from build123d import *

# Parameters (mm, degrees)
ESBO_O1_W                = 231.5
ESBO_O1_H                = 170
RESSALTO_EXTRUS_O1_DEPTH = 3
CORTE_EXTRUS_O1_REACH    = 145.639
ESBO_O2_W                = 17.807692308
ESBO_O2_H                = 6
CORTE_EXTRUS_O2_REACH    = 145.639
ESBO_O3_W                = 6
ESBO_O3_H                = 15.454545455


with BuildPart() as part:
    # Esboço1 → Ressalto-extrusão1 (new body)
    with BuildSketch(Plane(origin=(0, 0, 0), x_dir=(1, 0, 0), z_dir=(0, 1, 0))):
        Rectangle(ESBO_O1_W, ESBO_O1_H)
    extrude(amount=RESSALTO_EXTRUS_O1_DEPTH)

    # Esboço2 → Corte-extrusão1 (cut, up to next)
    with BuildSketch(Plane.XZ, mode=Mode.PRIVATE) as corte_extrus_o1_sk1:
        with Locations((-71.226153846, 82)):
            Rectangle(ESBO_O2_W, ESBO_O2_H)
    corte_extrus_o1_tool1 = extrude(corte_extrus_o1_sk1.sketch, amount=-CORTE_EXTRUS_O1_REACH, mode=Mode.PRIVATE) & part.part
    # Esboço2 → Corte-extrusão1 (cut, up to next)
    with BuildSketch(Plane.XZ, mode=Mode.PRIVATE) as corte_extrus_o1_sk2:
        with Locations((-106.846153846, 82)):
            Rectangle(ESBO_O2_W, ESBO_O2_H)
    corte_extrus_o1_tool2 = extrude(corte_extrus_o1_sk2.sketch, amount=-CORTE_EXTRUS_O1_REACH, mode=Mode.PRIVATE) & part.part
    # Esboço2 → Corte-extrusão1 (cut, up to next)
    with BuildSketch(Plane.XZ, mode=Mode.PRIVATE) as corte_extrus_o1_sk3:
        with Locations((-35.606153846, 82)):
            Rectangle(ESBO_O2_W, ESBO_O2_H)
    corte_extrus_o1_tool3 = extrude(corte_extrus_o1_sk3.sketch, amount=-CORTE_EXTRUS_O1_REACH, mode=Mode.PRIVATE) & part.part
    # Esboço2 → Corte-extrusão1 (cut, up to next)
    with BuildSketch(Plane.XZ, mode=Mode.PRIVATE) as corte_extrus_o1_sk4:
        with Locations((0.013846154, 82)):
            Rectangle(ESBO_O2_W, ESBO_O2_H)
    corte_extrus_o1_tool4 = extrude(corte_extrus_o1_sk4.sketch, amount=-CORTE_EXTRUS_O1_REACH, mode=Mode.PRIVATE) & part.part
    # Esboço2 → Corte-extrusão1 (cut, up to next)
    with BuildSketch(Plane.XZ, mode=Mode.PRIVATE) as corte_extrus_o1_sk5:
        with Locations((35.633846154, 82)):
            Rectangle(ESBO_O2_W, ESBO_O2_H)
    corte_extrus_o1_tool5 = extrude(corte_extrus_o1_sk5.sketch, amount=-CORTE_EXTRUS_O1_REACH, mode=Mode.PRIVATE) & part.part
    # Esboço2 → Corte-extrusão1 (cut, up to next)
    with BuildSketch(Plane.XZ, mode=Mode.PRIVATE) as corte_extrus_o1_sk6:
        with Locations((71.253846154, 82)):
            Rectangle(ESBO_O2_W, ESBO_O2_H)
    corte_extrus_o1_tool6 = extrude(corte_extrus_o1_sk6.sketch, amount=-CORTE_EXTRUS_O1_REACH, mode=Mode.PRIVATE) & part.part
    # Esboço2 → Corte-extrusão1 (cut, up to next)
    with BuildSketch(Plane.XZ, mode=Mode.PRIVATE) as corte_extrus_o1_sk7:
        with Locations((106.873846154, 82)):
            Rectangle(ESBO_O2_W, ESBO_O2_H)
    corte_extrus_o1_tool7 = extrude(corte_extrus_o1_sk7.sketch, amount=-CORTE_EXTRUS_O1_REACH, mode=Mode.PRIVATE) & part.part
    # Esboço2 → Corte-extrusão1 (cut, up to next)
    with BuildSketch(Plane.XZ, mode=Mode.PRIVATE) as corte_extrus_o1_sk8:
        with Locations((-71.226153846, -82)):
            Rectangle(ESBO_O2_W, ESBO_O2_H)
    corte_extrus_o1_tool8 = extrude(corte_extrus_o1_sk8.sketch, amount=-CORTE_EXTRUS_O1_REACH, mode=Mode.PRIVATE) & part.part
    # Esboço2 → Corte-extrusão1 (cut, up to next)
    with BuildSketch(Plane.XZ, mode=Mode.PRIVATE) as corte_extrus_o1_sk9:
        with Locations((-35.606153846, -82)):
            Rectangle(ESBO_O2_W, ESBO_O2_H)
    corte_extrus_o1_tool9 = extrude(corte_extrus_o1_sk9.sketch, amount=-CORTE_EXTRUS_O1_REACH, mode=Mode.PRIVATE) & part.part
    # Esboço2 → Corte-extrusão1 (cut, up to next)
    with BuildSketch(Plane.XZ, mode=Mode.PRIVATE) as corte_extrus_o1_sk10:
        with Locations((0.013846154, -82)):
            Rectangle(ESBO_O2_W, ESBO_O2_H)
    corte_extrus_o1_tool10 = extrude(corte_extrus_o1_sk10.sketch, amount=-CORTE_EXTRUS_O1_REACH, mode=Mode.PRIVATE) & part.part
    # Esboço2 → Corte-extrusão1 (cut, up to next)
    with BuildSketch(Plane.XZ, mode=Mode.PRIVATE) as corte_extrus_o1_sk11:
        with Locations((35.633846154, -82)):
            Rectangle(ESBO_O2_W, ESBO_O2_H)
    corte_extrus_o1_tool11 = extrude(corte_extrus_o1_sk11.sketch, amount=-CORTE_EXTRUS_O1_REACH, mode=Mode.PRIVATE) & part.part
    # Esboço2 → Corte-extrusão1 (cut, up to next)
    with BuildSketch(Plane.XZ, mode=Mode.PRIVATE) as corte_extrus_o1_sk12:
        with Locations((71.253846154, -82)):
            Rectangle(ESBO_O2_W, ESBO_O2_H)
    corte_extrus_o1_tool12 = extrude(corte_extrus_o1_sk12.sketch, amount=-CORTE_EXTRUS_O1_REACH, mode=Mode.PRIVATE) & part.part
    # Esboço2 → Corte-extrusão1 (cut, up to next)
    with BuildSketch(Plane.XZ, mode=Mode.PRIVATE) as corte_extrus_o1_sk13:
        with Locations((106.873846154, -82)):
            Rectangle(ESBO_O2_W, ESBO_O2_H)
    corte_extrus_o1_tool13 = extrude(corte_extrus_o1_sk13.sketch, amount=-CORTE_EXTRUS_O1_REACH, mode=Mode.PRIVATE) & part.part
    # Esboço2 → Corte-extrusão1 (cut, up to next)
    with BuildSketch(Plane.XZ, mode=Mode.PRIVATE) as corte_extrus_o1_sk14:
        with Locations((-106.846153846, -82)):
            Rectangle(ESBO_O2_W, ESBO_O2_H)
    corte_extrus_o1_tool14 = extrude(corte_extrus_o1_sk14.sketch, amount=-CORTE_EXTRUS_O1_REACH, mode=Mode.PRIVATE) & part.part
    add(corte_extrus_o1_tool1.solids().sort_by_distance((-71.226154, 0, 82))[0], mode=Mode.SUBTRACT)
    add(corte_extrus_o1_tool2.solids().sort_by_distance((-106.846154, 0, 82))[0], mode=Mode.SUBTRACT)
    add(corte_extrus_o1_tool3.solids().sort_by_distance((-35.606154, 0, 82))[0], mode=Mode.SUBTRACT)
    add(corte_extrus_o1_tool4.solids().sort_by_distance((0.013846, 0, 82))[0], mode=Mode.SUBTRACT)
    add(corte_extrus_o1_tool5.solids().sort_by_distance((35.633846, 0, 82))[0], mode=Mode.SUBTRACT)
    add(corte_extrus_o1_tool6.solids().sort_by_distance((71.253846, 0, 82))[0], mode=Mode.SUBTRACT)
    add(corte_extrus_o1_tool7.solids().sort_by_distance((106.873846, 0, 82))[0], mode=Mode.SUBTRACT)
    add(corte_extrus_o1_tool8.solids().sort_by_distance((-71.226154, 0, -82))[0], mode=Mode.SUBTRACT)
    add(corte_extrus_o1_tool9.solids().sort_by_distance((-35.606154, 0, -82))[0], mode=Mode.SUBTRACT)
    add(corte_extrus_o1_tool10.solids().sort_by_distance((0.013846, 0, -82))[0], mode=Mode.SUBTRACT)
    add(corte_extrus_o1_tool11.solids().sort_by_distance((35.633846, 0, -82))[0], mode=Mode.SUBTRACT)
    add(corte_extrus_o1_tool12.solids().sort_by_distance((71.253846, 0, -82))[0], mode=Mode.SUBTRACT)
    add(corte_extrus_o1_tool13.solids().sort_by_distance((106.873846, 0, -82))[0], mode=Mode.SUBTRACT)
    add(corte_extrus_o1_tool14.solids().sort_by_distance((-106.846154, 0, -82))[0], mode=Mode.SUBTRACT)

    # Esboço3 → Corte-extrusão2 (cut, up to next)
    with BuildSketch(Plane.XZ, mode=Mode.PRIVATE) as corte_extrus_o2_sk1:
        with Locations((112.75, 77.272727272)):
            Rectangle(ESBO_O3_W, ESBO_O3_H)
    corte_extrus_o2_tool1 = extrude(corte_extrus_o2_sk1.sketch, amount=-CORTE_EXTRUS_O2_REACH, mode=Mode.PRIVATE) & part.part
    # Esboço3 → Corte-extrusão2 (cut, up to next)
    with BuildSketch(Plane.XZ, mode=Mode.PRIVATE) as corte_extrus_o2_sk2:
        with Locations((-112.75, 77.272727272)):
            Rectangle(ESBO_O3_W, ESBO_O3_H)
    corte_extrus_o2_tool2 = extrude(corte_extrus_o2_sk2.sketch, amount=-CORTE_EXTRUS_O2_REACH, mode=Mode.PRIVATE) & part.part
    # Esboço3 → Corte-extrusão2 (cut, up to next)
    with BuildSketch(Plane.XZ, mode=Mode.PRIVATE) as corte_extrus_o2_sk3:
        with Locations((112.75, 46.362727273)):
            Rectangle(ESBO_O3_W, ESBO_O3_H)
    corte_extrus_o2_tool3 = extrude(corte_extrus_o2_sk3.sketch, amount=-CORTE_EXTRUS_O2_REACH, mode=Mode.PRIVATE) & part.part
    # Esboço3 → Corte-extrusão2 (cut, up to next)
    with BuildSketch(Plane.XZ, mode=Mode.PRIVATE) as corte_extrus_o2_sk4:
        with Locations((112.75, 15.452727273)):
            Rectangle(ESBO_O3_W, ESBO_O3_H)
    corte_extrus_o2_tool4 = extrude(corte_extrus_o2_sk4.sketch, amount=-CORTE_EXTRUS_O2_REACH, mode=Mode.PRIVATE) & part.part
    # Esboço3 → Corte-extrusão2 (cut, up to next)
    with BuildSketch(Plane.XZ, mode=Mode.PRIVATE) as corte_extrus_o2_sk5:
        with Locations((112.75, -15.457272728)):
            Rectangle(ESBO_O3_W, ESBO_O3_H)
    corte_extrus_o2_tool5 = extrude(corte_extrus_o2_sk5.sketch, amount=-CORTE_EXTRUS_O2_REACH, mode=Mode.PRIVATE) & part.part
    # Esboço3 → Corte-extrusão2 (cut, up to next)
    with BuildSketch(Plane.XZ, mode=Mode.PRIVATE) as corte_extrus_o2_sk6:
        with Locations((112.75, -46.367272728)):
            Rectangle(ESBO_O3_W, ESBO_O3_H)
    corte_extrus_o2_tool6 = extrude(corte_extrus_o2_sk6.sketch, amount=-CORTE_EXTRUS_O2_REACH, mode=Mode.PRIVATE) & part.part
    # Esboço3 → Corte-extrusão2 (cut, up to next)
    with BuildSketch(Plane.XZ, mode=Mode.PRIVATE) as corte_extrus_o2_sk7:
        with Locations((112.75, -77.277272728)):
            Rectangle(ESBO_O3_W, ESBO_O3_H)
    corte_extrus_o2_tool7 = extrude(corte_extrus_o2_sk7.sketch, amount=-CORTE_EXTRUS_O2_REACH, mode=Mode.PRIVATE) & part.part
    # Esboço3 → Corte-extrusão2 (cut, up to next)
    with BuildSketch(Plane.XZ, mode=Mode.PRIVATE) as corte_extrus_o2_sk8:
        with Locations((-112.75, 46.362727273)):
            Rectangle(ESBO_O3_W, ESBO_O3_H)
    corte_extrus_o2_tool8 = extrude(corte_extrus_o2_sk8.sketch, amount=-CORTE_EXTRUS_O2_REACH, mode=Mode.PRIVATE) & part.part
    # Esboço3 → Corte-extrusão2 (cut, up to next)
    with BuildSketch(Plane.XZ, mode=Mode.PRIVATE) as corte_extrus_o2_sk9:
        with Locations((-112.75, 15.452727273)):
            Rectangle(ESBO_O3_W, ESBO_O3_H)
    corte_extrus_o2_tool9 = extrude(corte_extrus_o2_sk9.sketch, amount=-CORTE_EXTRUS_O2_REACH, mode=Mode.PRIVATE) & part.part
    # Esboço3 → Corte-extrusão2 (cut, up to next)
    with BuildSketch(Plane.XZ, mode=Mode.PRIVATE) as corte_extrus_o2_sk10:
        with Locations((-112.75, -15.457272728)):
            Rectangle(ESBO_O3_W, ESBO_O3_H)
    corte_extrus_o2_tool10 = extrude(corte_extrus_o2_sk10.sketch, amount=-CORTE_EXTRUS_O2_REACH, mode=Mode.PRIVATE) & part.part
    # Esboço3 → Corte-extrusão2 (cut, up to next)
    with BuildSketch(Plane.XZ, mode=Mode.PRIVATE) as corte_extrus_o2_sk11:
        with Locations((-112.75, -46.367272728)):
            Rectangle(ESBO_O3_W, ESBO_O3_H)
    corte_extrus_o2_tool11 = extrude(corte_extrus_o2_sk11.sketch, amount=-CORTE_EXTRUS_O2_REACH, mode=Mode.PRIVATE) & part.part
    # Esboço3 → Corte-extrusão2 (cut, up to next)
    with BuildSketch(Plane.XZ, mode=Mode.PRIVATE) as corte_extrus_o2_sk12:
        with Locations((-112.75, -77.277272728)):
            Rectangle(ESBO_O3_W, ESBO_O3_H)
    corte_extrus_o2_tool12 = extrude(corte_extrus_o2_sk12.sketch, amount=-CORTE_EXTRUS_O2_REACH, mode=Mode.PRIVATE) & part.part
    add(corte_extrus_o2_tool1.solids().sort_by_distance((112.75, 0, 77.272727))[0], mode=Mode.SUBTRACT)
    add(corte_extrus_o2_tool2.solids().sort_by_distance((-112.75, 0, 77.272727))[0], mode=Mode.SUBTRACT)
    add(corte_extrus_o2_tool3.solids().sort_by_distance((112.75, 0, 46.362727))[0], mode=Mode.SUBTRACT)
    add(corte_extrus_o2_tool4.solids().sort_by_distance((112.75, 0, 15.452727))[0], mode=Mode.SUBTRACT)
    add(corte_extrus_o2_tool5.solids().sort_by_distance((112.75, 0, -15.457273))[0], mode=Mode.SUBTRACT)
    add(corte_extrus_o2_tool6.solids().sort_by_distance((112.75, 0, -46.367273))[0], mode=Mode.SUBTRACT)
    add(corte_extrus_o2_tool7.solids().sort_by_distance((112.75, 0, -77.277273))[0], mode=Mode.SUBTRACT)
    add(corte_extrus_o2_tool8.solids().sort_by_distance((-112.75, 0, 46.362727))[0], mode=Mode.SUBTRACT)
    add(corte_extrus_o2_tool9.solids().sort_by_distance((-112.75, 0, 15.452727))[0], mode=Mode.SUBTRACT)
    add(corte_extrus_o2_tool10.solids().sort_by_distance((-112.75, 0, -15.457273))[0], mode=Mode.SUBTRACT)
    add(corte_extrus_o2_tool11.solids().sort_by_distance((-112.75, 0, -46.367273))[0], mode=Mode.SUBTRACT)
    add(corte_extrus_o2_tool12.solids().sort_by_distance((-112.75, 0, -77.277273))[0], mode=Mode.SUBTRACT)


solid = part.part
For this review, take the finished solid that the model builds, in its own axes (mm). Give positions to 0.01 mm unless a question says otherwise; leave off trailing zeros. Order: outer loops, then holes, each group sorted by start corner. A loop starts at its lowest first (then second) coordinate and runs counter-clockwise, first axis right, second up. Notation, with made-up numbers: M -24,-27 L -5,-27 A29 ccw -5,3 Z; hole C 21.25,-4 d8. An arc over 180 degrees is marked long. Answer in a Markdown table with one row per item. Add a question column.
(1) For pin 1 (1.5 mm diameter, centred on x = -111.5, y = 1.5, fed in from +Z); pin 2 (1.5 mm diameter, centred on x = -70.5, y = 1, fed in from +Z); pin 3 (0.9 mm diameter, centred on x = -113, y = 2, fed in from -Z), all flat-tipped, find the tip position at first contact; note any pin that passes through.
(2) Wall thickness on probe 1 along Z at (x, y) = (-67, 1.95); probe 2 along X at (y, z) = (0.3, -48): over which ranges is each line inside the solid? List them lowest first. Write a range as [from, to].
(3) Consider section B-B on z = 73.5. State the section outline as (x, y) points.
(4) Consider section A-A on x = -5. State the section outline as (y, z) points, and give its area (3 significant figures).
Evaluation:
| question | item | result |
|---|---|---|
| 1 | pin 1 | stops at z = 69.55 |
| 1 | pin 2 | stops at z = 79 |
| 1 | pin 3 | stops at z = -69.55 |
| 2 | probe 1 | z = [-79, 79] |
| 2 | probe 2 | x = [-109.75, 109.75] |
| 3 | outline | M -109.75,0 L 109.75,0 L 109.75,3 L -109.75,3 Z |
| 4 | outline | M 0,-79 L 3,-79 L 3,79 L 0,79 Z |
| 4 | area | 474 mm^2 |
